```python
from build123d import *

# Parameters (mm, degrees)
CROQUIS1_W              = 90
CROQUIS1_H              = 80
CROQUIS1_R              = 28.9
SALIENTE_EXTRUIR1_DEPTH = 5
CROQUIS2_R              = 28.9
CROQUIS2_R_2            = 23.25
SALIENTE_EXTRUIR2_DEPTH = 3
CROQUIS4_W              = 10
CROQUIS4_H              = 25
CORTAR_EXTRUIR2_DEPTH   = 62.032778079
CHAFL_N2_SIZE           = 7.5
CROQUIS9_R              = 2.5
CORTAR_EXTRUIR3_DEPTH   = 10


with BuildPart() as part:
    # Croquis1 → Saliente-Extruir1 (new, symmetric)
    with BuildSketch(Plane.XY):
        Rectangle(CROQUIS1_W, CROQUIS1_H)
        Circle(CROQUIS1_R, mode=Mode.SUBTRACT)
    extrude(amount=SALIENTE_EXTRUIR1_DEPTH, both=True)

    # Croquis2 → Saliente-Extruir2 (add)
    with BuildSketch(Plane(origin=(0, 0, -5), x_dir=(-1, 0, 0), z_dir=(0, 0, -1))):
        Circle(CROQUIS2_R)
        Circle(CROQUIS2_R_2, mode=Mode.SUBTRACT)
    extrude(amount=-SALIENTE_EXTRUIR2_DEPTH)

    # Croquis4 → Cortar-Extruir2 (cut, through all)
    with BuildSketch(Plane.XY.offset(5)):
        with Locations((-45, 0)):
            Rectangle(CROQUIS4_W, CROQUIS4_H)
        with Locations((45, 0)):
            Rectangle(CROQUIS4_W, CROQUIS4_H)
    extrude(amount=-CORTAR_EXTRUIR2_DEPTH, mode=Mode.SUBTRACT)

    # Chaflán2
    chafl_n2_edges = [part.edges().sort_by_distance(p)[0] for p in [
        (45, -40, 0),
        (-45, -40, 0),
        (-45, 40, 0),
        (45, 40, 0),
    ]]
    chamfer(chafl_n2_edges, length=CHAFL_N2_SIZE)

    # Croquis9 → Cortar-Extruir3 (cut)
    with BuildSketch(Plane.XZ.offset(40)):
        with Locations(Location((-25, 0, 0), (0, 0, 270))):
            Circle(CROQUIS9_R)
        with Locations(Location((25, 0, 0), (0, 0, 270))):
            Circle(CROQUIS9_R)
    cortar_extruir3 = extrude(amount=-CORTAR_EXTRUIR3_DEPTH, mode=Mode.SUBTRACT)

    # Simetría1: Cortar-Extruir3 across plane
    add(cortar_extruir3.mirror(Plane.ZX), mode=Mode.SUBTRACT)


solid = part.part
```
Model file for the job. Use its own axes, mm. A direction names the side the tool comes from. Give positions to 0.01 mm unless a question says otherwise; leave off trailing zeros. Loops run counter-clockwise (first coordinate to the right, second up) from the corner with the lowest first, then second, coordinate; pieces in that order, holes last. Notation, with made-up numbers: (-10.75, 43) -> (6.25, 43) arc R26 cw to (6.25, 70) -> close; hole circle Ø4 at (-19.5, -18.75). An arc over 180 degrees is marked (long way). Use CSV: the item, a comma, the result in double quotes. Start each with the question number.
1) Slice it at A-A on y = 0. Give the cut face in (x, z).
2) Tool access for faces 1 (the flat face through (40, 0, 0)), 2 (the cylindrical face through (27.48, -35.07, 0.33)), 3 (the flat face through (-2, 24, -2)): list every direction of +Z, -Z, +X, -X, +Y, -Y with a clear straight run to the whole face (end or side of a thin tool).
3) Slice it at D-D on y = 35. Give the cut face in (x, z), plus the area to 3 significant figures.
4) Wall check: line 1 (X direction, y = 32.25, z = 0); line 2 (X direction, y = 32.75, z = 0); line 3 (Y direction, x = -4.5, z = -1.75). Give the ranges that are in metal, low to high.
5) Flat gauge pins, fed straight in: pin 1 Ø4 at (x, z) = (42, 1.5) entering from -Y; pin 2 Ø1.5 at (x, z) = (-26, -0.5) entering from -Y; pin 3 Ø2.5 at (x, z) = (42, 1) entering from +Y. Where does each tip first touch, or does it go through?
6) Mould opens along X. For faces 4 (the flat face through (-41.3, 36.2, 0.1)), 5 (the flat face through (-19, 18, -5)), 6 (the cylindrical face through (-22.52, 35.07, 0.33)), 7 (the flat face through (25, 30, 0)) say: released by +X, released by -X, zero draft, split by the parting line, or undercut.
Computed values:
1,outline,"(-40, -5) -> (-23.25, -5) -> (-23.25, -2) -> (-28.9, -2) -> (-28.9, 5) -> (-40, 5) -> close; (23.25, -5) -> (40, -5) -> (40, 5) -> (28.9, 5) -> (28.9, -2) -> (23.25, -2) -> close"
2,face 1,"+Z, -Z, +X"
2,face 2,"-Y"
2,face 3,"+Z"
3,outline,"(-42.5, -5) -> (42.5, -5) -> (42.5, 5) -> (-42.5, 5) -> close; hole circle Ø5 at (-25, 0); hole circle Ø5 at (25, 0)"
3,area,"811 mm^2"
4,line 1,"x = -45 to -27.5, -22.5 to 22.5, 27.5 to 45"
4,line 2,"x = -44.75 to -27.5, -22.5 to 22.5, 27.5 to 44.75"
4,line 3,"y = -40 to -28.55, 28.55 to 40"
5,pin 1,"stops at y = -37.5"
5,pin 2,"stops at y = -30"
5,pin 3,"stops at y = 36.75"
6,face 4,"released by -X"
6,face 5,"zero draft"
6,face 6,"undercut"
6,face 7,"undercut"
